Geometry: see drawing. Coordinates: mm, zero at the bounding-box minimum. A direction names the side the tool comes from. Round coordinates to 2 decimals unless told otherwise and drop trailing zeros. Loops run counter-clockwise (first coordinate to the right, second up) from the corner with the lowest first, then second, coordinate; pieces in that order, holes last. Notation, with made-up numbers: (4, 23.5) -> (60, 23.5) arc R29 cw to (60, 50.5) -> close; hole circle Ø1 at (37.25, -27). An arc over 180 degrees is marked (long way). Answer in a Markdown table with one row per item.
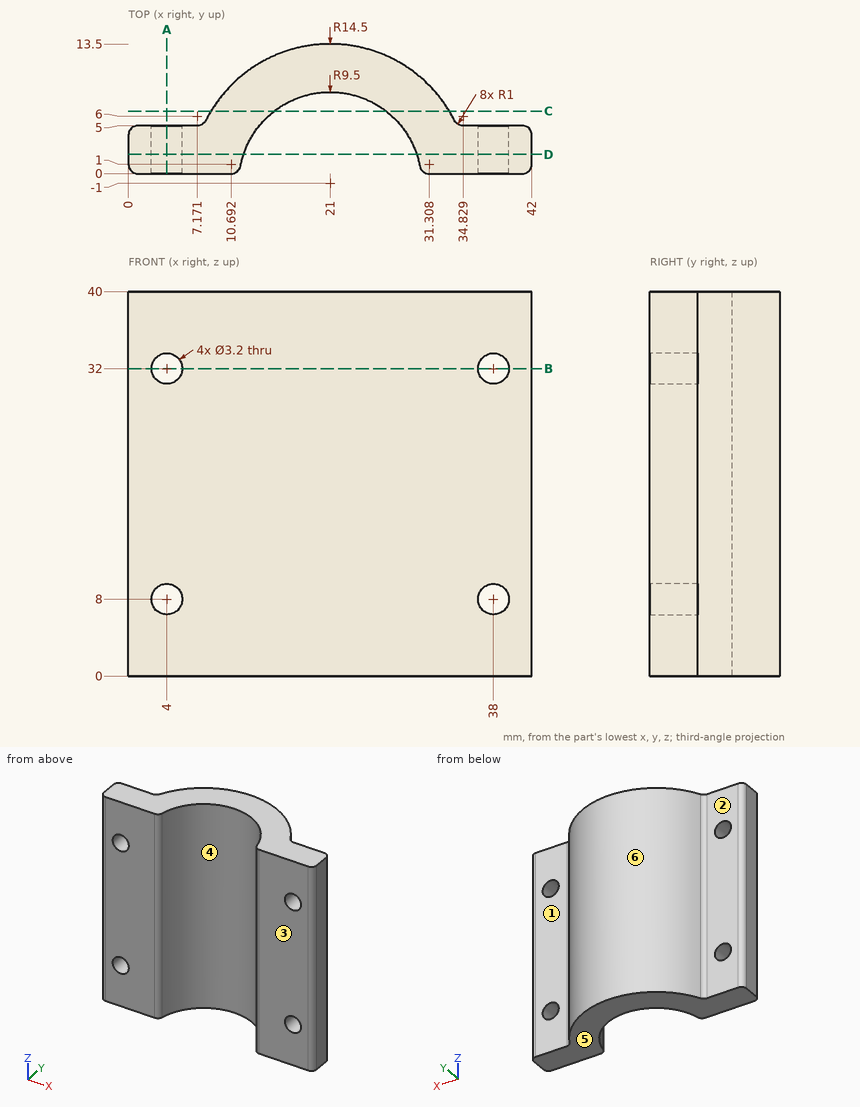
Item 1: Section query A-A, the plane x = 4. Output: boundary loops of the cut face in (y, z).
Ans:
| item | result |
|---|---|
| outline | (0, 0) -> (5, 0) -> (5, 6.4) -> (0, 6.4) -> close; (0, 9.6) -> (5, 9.6) -> (5, 30.4) -> (0, 30.4) -> close; (0, 33.6) -> (5, 33.6) -> (5, 40) -> (0, 40) -> close |
Item 2: Mould query, pull axis X, two halves, no side actions, for the marked faces 4, 5 and 6. Classes: released by +X, released by -X, zero draft, split by the parting line, or undercut.
Ans:
| item | result |
|---|---|
| face 4 | undercut |
| face 5 | zero draft |
| face 6 | split by the parting line |
Item 3: Ray query, L1, parallel to X at y = 3.35, z = 8 (1 decimal); L2, parallel to X at y = 1.25, z = 8; L3, parallel to Y at x = 2, z = 9.5. Return the intervals inside material, ascending.
Ans:
| item | result |
|---|---|
| L1 | 0 to 2.4, 5.6 to 12.6, 29.4 to 36.4, 39.6 to 42 |
| L2 | 0 to 2.4, 5.6 to 11.77, 30.23 to 36.4, 39.6 to 42 |
| L3 | 0 to 5 |
Item 4: Section query C-C, the plane y = 6.5. Output: boundary loops of the cut face in (x, z).
Ans:
| item | result |
|---|---|
| outline | (8.59, 0) -> (15.17, 0) -> (15.17, 40) -> (8.59, 40) -> close; (26.83, 0) -> (33.41, 0) -> (33.41, 40) -> (26.83, 40) -> close |
Item 5: Section query D-D, the plane y = 2. Output: boundary loops of the cut face in (x, z), and give its area (3 significant figures).
Ans:
| item | result |
|---|---|
| outline | (0, 0) -> (11.99, 0) -> (11.99, 40) -> (0, 40) -> close; (30.01, 0) -> (42, 0) -> (42, 40) -> (30.01, 40) -> close; hole circle Ø3.2 at (4, 8); hole circle Ø3.2 at (4, 32); hole circle Ø3.2 at (38, 8); hole circle Ø3.2 at (38, 32) |
| area | 927 mm2 |
Item 6: First-contact query: P1, Ø3, axis at x = 4, z = 20, coming from the +Y side; P2, Ø3, axis at x = 18.5, z = 16.5, coming from the +Y side; P3, Ø3, axis at x = 38, z = 32, coming from the -Y side; P4, Ø10, axis at x = 28, z = 16, coming from the +Y side. Flat tips, straight axial feed; report the tip coordinate or a pass-through.
Ans:
| item | result |
|---|---|
| P1 | y = 5 |
| P2 | y = 13.47 |
| P3 | through |
| P4 | y = 13.36 |
Item 7: Section query B-B, the plane z = 32. Output: boundary loops of the cut face in (x, y).
Ans:
| item | result |
|---|---|
| outline | (0, 1) arc R1 ccw to (1, 0) -> (2.4, 0) -> (2.4, 5) -> (1, 5) arc R1 ccw to (0, 4) -> close; (5.6, 0) -> (10.69, 0) arc R1 ccw to (11.67, 0.81) arc R9.5 cw to (30.33, 0.81) arc R1 ccw to (31.31, 0) -> (36.4, 0) -> (36.4, 5) -> (34.83, 5) arc R1 cw to (33.94, 5.55) arc R14.5 ccw to (8.06, 5.55) arc R1 cw to (7.17, 5) -> (5.6, 5) -> close; (39.6, 0) -> (41, 0) arc R1 ccw to (42, 1) -> (42, 4) arc R1 ccw to (41, 5) -> (39.6, 5) -> close |
Item 8: Set-up query: the marked faces 1, 2 and 3. Return all of +Z, -Z, +X, -X, +Y, -Y with unobstructed straight access to the full face (end or side cutting, diameter ignored); none if empty.
Ans:
| item | result |
|---|---|
| face 1 | +Z, -Z, +X, +Y |
| face 2 | +Z, -Z, -X, +Y |
| face 3 | +Z, -Z, +X, -X, -Y |
